Autodesk Fusion 360 part; units mm, degrees
sketch "Sketch1" plane through (0, 0, 0) normal (0, 0, 1) x (1, 0, 0)
  line L0 (0, 198.4375) -> (111.125, 198.4375)
  line L1 (111.125, 198.4375) -> (111.125, 0)
  line L2 (111.125, 198.4375) -> (89.6938, 198.4375)
  circle A0 centre (75.9063, 180.1813) radius 1
  circle A1 centre (90.1938, 180.1813) radius 1
  circle A2 centre (20.4312, 180.1813) radius 1
  circle A3 centre (34.7188, 180.1813) radius 1
  line L3 (111.125, 198.4375) -> (80.962, 198.4375)
  line L4 (80.962, 198.4375) -> (80.962, 192.0875)
  line L5 (111.125, 0) -> (104.775, 0)
  line L6 (0, 0) -> (111.125, 0)
  circle A4 centre (14.0812, 15.0813) radius 1
  circle A5 centre (28.3687, 15.0813) radius 1
  circle A6 centre (75.4062, 15.0813) radius 1
  circle A7 centre (90.1937, 15.0813) radius 1
  circle A8 centre (7.3495, 15.2875) radius 1.5
  circle A9 centre (99.0125, 15.2875) radius 1.5
  line L7 (80.962, 144.4625) -> (80.962, 150.8125)
  line L8 (80.962, 150.8125) -> (61.912, 150.8125)
  line L9 (61.912, 150.8125) -> (61.912, 144.4625)
  line L10 (80.962, 198.4375) -> (80.962, 192.0875)
  line L11 (80.962, 192.0875) -> (61.912, 192.0875)
  line L12 (61.912, 192.0875) -> (61.912, 198.4375)
  line L13 (0, 0) -> (0, 198.4375)
  line L14 (0, 141.2875) -> (111.125, 141.2875)
  line L15 (61.912, 144.4625) -> (0, 144.4625)
  line L16 (80.962, 144.4625) -> (111.125, 144.4625)
  dimension "d1" = 111.125
  dimension "d2" = 198.4375
  dimension "d3" = 111.125
  dimension "d39" = 14.2875
  dimension "d49" = 6.35
extrude "Extrude18" add sketch "Sketch1" along normal blind 3.175 contours L0 L1 L2 L3 L4 L7 L8 L9 L10 L11 L12 L13 L15 L16 makes body 1
extrude "Extrude19" add sketch "Sketch1" along normal blind 3.175 separate body contours L1 L5 L6 L13 L14 makes body 2
extrude "Extrude20" add sketch "Sketch1" along normal blind 57.15 contours L1 L7 L8 L9 L13 L14 L15 L16 bodies 1 2
extrude "Extrude21" add sketch "Sketch1" along normal blind 57.15 contours L0 L4 L10 L11 L12 bodies 1
sketch "Sketch5" plane through (0, 0, 3.175) normal (0, 0, 1) x (-1, 0, 0)
  circle A0 centre (-28.3687, -15.0813) radius 1
  circle A1 centre (-99.0125, -15.2875) radius 1.5
  circle A2 centre (-7.3495, -15.2875) radius 1.5
  circle A3 centre (-90.1937, -15.0813) radius 1
  circle A4 centre (-75.4062, -15.0813) radius 1
  circle A5 centre (-14.0812, -15.0813) radius 1
  line L0 (0, 0) -> (-111.125, 0)
  line L1 (-111.125, 0) -> (-111.125, -141.2875)
  line L2 (-111.125, -141.2875) -> (0, -141.2875)
  line L3 (0, -141.2875) -> (0, 0)
  circle A6 centre (-7.3495, -15.2875) radius 2.5
  circle A7 centre (-99.0125, -15.2875) radius 2.5
  circle A8 centre (-99.0125, -73.2312) radius 1.5
  circle A9 centre (-7.3495, -73.2312) radius 1.5
  dimension "d170" = 1
  dimension "d171" = 1
  dimension "d219" = 3
extrude "Extrude24" add sketch "Sketch5" along normal blind 6.35 contours A6 bodies 1
extrude "Extrude25" add sketch "Sketch5" along normal blind 6.35 contours A7 bodies 1
sketch "Sketch6" plane through (61.912, 0, 0) normal (-1, 0, 0) x (0, -1, 0)
  line L0 (-150.8125, 3.175) -> (-144.4625, 3.175)
  line L1 (-144.4625, 3.175) -> (-144.4625, 57.15)
  line L2 (-144.4625, 57.15) -> (-150.8125, 57.15)
  line L3 (-150.8125, 57.15) -> (-150.8125, 3.175)
  circle A0 centre (-196.0563, 52.3875) radius 1.25
  circle A1 centre (-196.0563, 42.8625) radius 1.25
  circle A2 centre (-146.8433, 52.3875) radius 1.25
  circle A3 centre (-146.8433, 42.8625) radius 1.25
extrude "Extrude26" cut sketch "Sketch6" against normal blind 19.05 contours A0 bodies 1
extrude "Extrude27" cut sketch "Sketch6" against normal blind 19.05 contours A1 | A2 | A3 bodies 1
extrude "Extrude28" cut 1 faces at (80.962, 195.4959, 15.9887) along direction (-1, 0, 0) blind 6.35 on bodies 1 bodies 1
extrude "Extrude29" cut 1 faces at (80.962, 147.4039, 15.9887) along direction (-1, 0, 0) blind 6.35 on bodies 1 bodies 1
sketch "Sketch7" plane through (0, 0, 57.15) normal (0, 0, 1) x (-1, 0, 0)
  line L0 (-74.612, -144.4625) -> (-74.612, -150.8125)
  line L1 (-74.612, -150.8125) -> (-61.912, -150.8125)
  line L2 (-61.912, -150.8125) -> (-61.912, -144.4625)
  line L3 (-61.912, -144.4625) -> (0, -144.4625)
  line L4 (0, -144.4625) -> (0, -141.2875)
  line L5 (0, -141.2875) -> (-111.125, -141.2875)
  line L6 (-111.125, -141.2875) -> (-111.125, -144.4625)
  line L7 (-74.612, -144.4625) -> (-74.612, -143.4625)
  line L8 (-74.612, -143.4625) -> (-94.612, -143.4625)
  line L9 (-94.612, -143.4625) -> (-94.612, -144.4625)
  line L10 (-74.612, -144.4625) -> (-94.612, -144.4625)
  dimension "d208" = 20
extrude "Extrude32" cut sketch "Sketch7" against normal blind 54 bodies 1
extrude "Extrude34" cut 1 faces at (62.1192, 99.547, 3.175) along direction (0, 0, -1) blind 14 on bodies 1 bodies 1 makes body 3 at (4.8526, 15.4121, 6.35) makes body 4 at (74.0833, 141.2875, 38.1)
extrude "Extrude35" add sketch "Sketch5" against normal blind 3.175 contours L0 L1 L2 L3 bodies 1 3 4
sketch "Sketch8" plane through (0, 0, 3.175) normal (0, 0, 1) x (-1, 0, 0)
  circle A0 centre (-7.3495, -73.2312) radius 1.5
  circle A1 centre (-99.0125, -15.2875) radius 2.5
  circle A2 centre (-28.3687, -15.0813) radius 1
  circle A3 centre (-75.4062, -15.0813) radius 1
  circle A4 centre (-14.0812, -15.0813) radius 1
  circle A5 centre (-90.1937, -15.0813) radius 1
  circle A6 centre (-7.3495, -15.2875) radius 2.5
  circle A7 centre (-99.0125, -73.2312) radius 1.5
  line L0 (0, -141.2875) -> (0, 0)
  line L1 (0, 0) -> (-111.125, 0)
  line L2 (-111.125, 0) -> (-111.125, -141.2875)
  line L3 (-111.125, -141.2875) -> (0, -141.2875)
  circle A8 centre (-7.3495, -73.2312) radius 2.5
  circle A9 centre (-99.0125, -73.2312) radius 2.5
  dimension "d226" = 1
  dimension "d227" = 1
extrude "Extrude36" add sketch "Sketch8" along normal blind 6.35 contours A8 | A9 bodies 1
sketch "Sketch9" plane through (0, 144.4625, 0) normal (0, 1, 0) x (-1, 0, 0)
  line L0 (-61.912, 3.175) -> (0, 3.175)
  line L1 (0, 3.175) -> (0, 57.15)
  line L2 (0, 57.15) -> (-61.912, 57.15)
  line L3 (-61.912, 57.15) -> (-61.912, 3.175)
  line L4 (-111.125, 57.15) -> (-94.6, 57.15)
  line L5 (-111.125, 57.15) -> (-102.8625, 57.15)
  line L6 (-111.125, 3.175) -> (-111.125, 20.875)
  line L7 (-111.125, 20.875) -> (-102.862, 20.875)
  circle A0 centre (-102.862, 20.875) radius 2.5
  line L8 (0, 3.175) -> (0, 20.875)
  line L9 (0, 20.875) -> (-8.263, 20.875)
  circle A1 centre (-8.263, 20.875) radius 2.5
  dimension "d247" = 17.7
  dimension "d248" = 8.263
  dimension "d249" = 5
  dimension "d250" = 17.7
  dimension "d253" = 5
extrude "Extrude40" cut sketch "Sketch9" against normal blind 10 contours A1 | A0 bodies 1
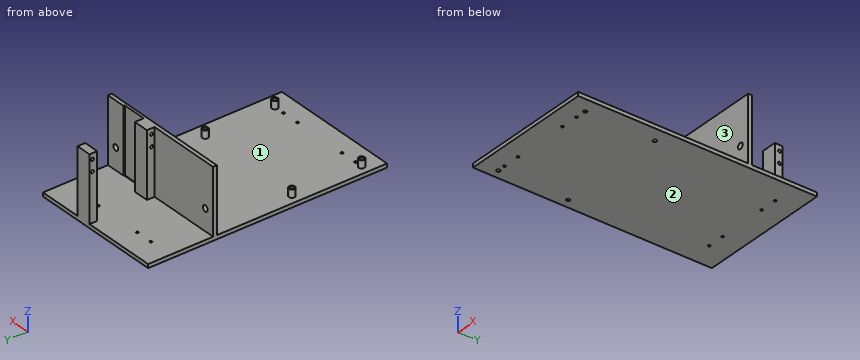
Input: part model. Units: mm. Frame: model coordinates. Face numbers are marked on the shaded views. Give positions to 0.01 mm unless a question says otherwise; leave off trailing zeros. Write each loop counter-clockwise with the first axis right and the second up, starting at its lowest first coordinate (ties: lowest second). Pieces come first, ordered by that corner, then holes.
Q1. Material intervals for probe 1 along Z at (x, y) = (39, 123.5) (3 decimals); probe 2 along Y at (x, z) = (88.5, 26); probe 3 along Y at (x, z) = (55, 52.5), sorted ascending.
Q2. Section C-C, the plane y = 105.5. Output: boundary loops of the cut face in (x, z) (3 decimals), plus the area to 3 significant figures.
Q3. Section A-A, the plane z = 34.5. Output: boundary loops of the cut face in (x, y) (1 decimal), plus the area to 3 significant figures.
Q4. First-contact query: P1, Ø4, axis at x = 99.01, y = 73.23, coming from the +Z side (3 decimals); P2, Ø4, axis at y = 196.06, z = 52.39, coming from the -X side; P3, Ø4, axis at x = 70.5, z = 38.5, coming from the -Y side; P4, Ø1.2, axis at x = 75.91, y = 180.18, coming from the -Z side. Flat tips, straight axial feed; report the tip coordinate or a pass-through.
Q5. Pull-direction query (Z, two-part tool) for the marked faces 1, 2 and 3; classes: pulls with the +Z half, pulls with the -Z half, needs draft (parallel to the pull), parting line crosses it, or undercut.
Filled in:
1. probe 1: z = 0 to 3.175
1. probe 2: y = 141.29 to 143.46
1. probe 3: y = 141.29 to 144.46
2. outline: (0, 0) - (111.125, 0) - (111.125, 3.175) - (0, 3.175) - close
2. area: 353 mm2
3. outline: (0, 141.3) - (111.1, 141.3) - (111.1, 144.5) - (94.6, 144.5) - (94.6, 143.5) - (74.6, 143.5) - (74.6, 150.8) - (61.9, 150.8) - (61.9, 144.5) - (0, 144.5) - close; (61.9, 192.1) - (74.6, 192.1) - (74.6, 198.4) - (61.9, 198.4) - close
3. area: 494 mm2
4. P1: stops at z = 9.525
4. P2: stops at x = 61.91
4. P3: stops at y = 141.29
4. P4: passes through
5. face 1: pulls with the +Z half
5. face 2: pulls with the -Z half
5. face 3: needs draft
